Autodesk Inventor part; units mm, degrees
ref_plane "YZ Plane" through (0, 0, 0) normal (1, 0, 0) x (0, 1, 0)
ref_plane "XZ Plane" through (0, 0, 0) normal (0, 1, 0) x (-1, 0, 0)
ref_plane "XY Plane" through (0, 0, 0) normal (0, 0, 1) x (1, 0, 0)
sketch "Szkic1" plane through (0, 0, 0) normal (0, 1, 0) x (-1, 0, 0)
  line L0 (0, 0) -> (0, -135)
  line L1 (0, 0) -> (-135, 0)
  arc A0 (-10, -125) -> (0, -135) centre (0, -125) ccw
  arc A1 (-135, 0) -> (-125, -10) centre (-125, 0) ccw
  arc A2 (-10, -125) -> (-125, -10) centre (-125, -125) ccw
  line L2 (0, 0) -> (135, 0)
  arc A3 (0, -135) -> (10, -125) centre (0, -125) ccw
  arc A4 (125, -10) -> (135, 0) centre (125, 0) ccw
  arc A5 (125, -10) -> (10, -125) centre (125, -125) ccw
  line L3 (0, 0) -> (0, 135)
  arc A6 (0, 135) -> (-10, 125) centre (0, 125) ccw
  arc A7 (-125, 10) -> (-135, 0) centre (-125, 0) ccw
  arc A8 (-125, 10) -> (-10, 125) centre (-125, 125) ccw
  arc A9 (10, 125) -> (0, 135) centre (0, 125) ccw
  arc A10 (135, 0) -> (125, 10) centre (125, 0) ccw
  arc A11 (10, 125) -> (125, 10) centre (125, 125) ccw
  circle A12 centre (-127, 0) radius 2.5
  circle A13 centre (-76, 0) radius 2.5
  circle A14 centre (0, 127) radius 2.5
  circle A15 centre (0, 76) radius 2.5
  circle A16 centre (0, -127) radius 2.5
  circle A17 centre (0, -76) radius 2.5
  circle A18 centre (127, 0) radius 2.5
  circle A19 centre (76, 0) radius 2.5
  dimension "d13" = 135
  dimension "d14" = 135
  dimension "d15" = 20
  dimension "d16" = 20
  dimension "d17" = 115
  dimension "d18" = 125
  dimension "sruba" = 5
  dimension "d20" = 8
  dimension "d21" = 5
  dimension "d22" = 51
  dimension "d23" = 5
  dimension "d24" = 5
  dimension "d25" = 8
  dimension "d26" = 51
extrude "Wyciągnięcie proste1" add sketch "Szkic1" along normal blind 3.74
sketch "Szkic2" plane through (0, 0, 0) normal (0, -1, 0) x (1, 0, 0)
  arc A0 (-10, -125) -> (10, -125) centre (0, -125) ccw
  circle A1 centre (-127, 0) radius 2.5
  circle A2 centre (-76, 0) radius 2.5
  circle A3 centre (76, 0) radius 2.5
  circle A4 centre (127, 0) radius 2.5
  circle A5 centre (0, -76) radius 2.5
  circle A6 centre (0, 76) radius 2.5
  circle A7 centre (0, 127) radius 2.5
  circle A8 centre (0, -127) radius 2.5
  point P0 (0, 0)
hole "Otwór1" at (0, 0, 127) at (0, 0, 76) at (-127, 0, 0) at (-76, 0, 0) at (0, 0, -76) at (0, 0, -125) at (76, 0, 0) at (127, 0, 0) direction (0, 1, 0) diameter 5 depth 8 tip angle 118
equation "\"d14\" = d13"
equation "\"d16\" = d15"
equation "\"d21\" = sruba"
equation "\"d23\" = sruba"
equation "\"d24\" = sruba"
equation "\"d25\" = d20"
equation "\"d26\" = d22"
equation "\"d27\" = sruba"
properties part number "Podstawa" material "Tworzywo sztuczne ABS"
Verification items for the finished model (mm, model axes). Give positions to 0.01 mm unless a question says otherwise; leave off trailing zeros. Loops run counter-clockwise (first coordinate to the right, second up) from the corner with the lowest first, then second, coordinate; pieces in that order, holes last. Notation, with made-up numbers: (-38, -13) - (-6, -13) arc R13 cw to (-6, -5) - close; hole circle Ø9 at (67, -10). An arc over 180 degrees is marked (long way). Write item = value, one per line. Start each with the question number.
Q1. Thickness scan on line 1 (X direction, y = 1.7, z = 0); line 2 (Z direction, x = -127, y = 1.5); line 3 (X direction, y = 2.1, z = -76). Record the ranges inside material, lowest first.
Q2. Cross-section at A-A, the plane y = 1.45. State how many separate pieces and enclosed holes the cut face has, and give its area (3 significant figures).
Q3. Cross-section at B-B, the plane z = -82. Enter the section's corners in (x, y), and give its area (3 significant figures).
Q4. Cross-section at C-C, the plane x = -31. Enter the section's corners in (y, z).
Q5. Depth check by flat-ended pin: P1, Ø1.5, axis at x = -40, y = 1.5, coming from the -Z side; P2, Ø1.5, axis at y = 2.5, z = -36, coming from the -X side. Enter the tip coordinate at first touch or a pass-through.
Answer key:
q1.line_1 = -135 to -129.5, -124.5 to -78.5, -73.5 to 73.5, 78.5 to 124.5, 129.5 to 135
q1.line_2 = -9.8 to -2.5, 2.5 to 9.8
q1.line_3 = -20.96 to -2.5, 2.5 to 20.96
q2.separate_pieces = 1
q2.enclosed_holes = 8
q2.area = 21,400 mm^2
q3.outline = (-18.34, 0) - (18.34, 0) - (18.34, 3.74) - (-18.34, 3.74) - close
q3.area = 137 mm^2
q4.outline = (0, -58.75) - (3.74, -58.75) - (3.74, 58.75) - (0, 58.75) - close
q5.P1 = -48.37
q5.P2 = -53.1
